Here's how the part is built. I have some questions about the finished solid (model axes, mm). A direction names the side the tool comes from. Give positions to 0.01 mm unless a question says otherwise; leave off trailing zeros. Loops run counter-clockwise (first coordinate to the right, second up) from the corner with the lowest first, then second, coordinate; pieces in that order, holes last.
Q1. Suppose I cut it at B-B (y = 81). List the corners of the cut face in (x, z) for me, and give its area (3 significant figures).
Q2. Suppose I cut it at A-A (y = 19). List the corners of the cut face in (x, z) for me, and give its area (3 significant figures).
Q3. I need wall thicknesses on probe 1 along Y at (x, z) = (3.25, -1.75); probe 2 along Y at (x, z) = (4.25, -3.5) (3 decimals); probe 3 along Z at (x, y) = (0.5, 37.5). Which ranges of each line are inside material? Lowest first, please.
Q4. Thinking about a two-plate mould opening in Z: for faces 4 (the face through (3.493, 83.161, 0.593)), 5 (the face through (3, 20, -6.983)), 6 (the face through (3, 20, 1.017)), 7 (the face through (3.04, 33, -8.75)), which applies, pulls with the +Z half, pulls with the -Z half, needs draft (parallel to the pull), parting line crosses it, or undercut?
Q5. Suppose I cut it at C-C (y = 59.5). List the corners of the cut face in (x, z) for me, and give its area (3 significant figures).
Q6. For faces 1 (the face through (7, 98, -6.755)), 2 (the face through (3, 28.943, -3)), 3 (the face through (7, 98, 0.789)), which set-ups out of +Z, -Z, +X, -X, +Y, -Y let a thin tool reach every point of the face, with its end or its side?
Q7. I'm going to push flat-ended pins straight in: P1, Ø4, axis at y = 77, z = -6, coming from the -X side; P2, Ø2.5, axis at y = 105.83, z = -2.98, coming from the -X side; P3, Ø1.8, axis at x = 3, z = -3, coming from the +Y side; P4, Ø4, axis at x = 5.5, y = 96.5, coming from the +Z side. Where does each tip first touch, or does it pass through?
```python
from build123d import *

# Parameters (mm, degrees)
SKETCH1_R               = 10
SKETCH1_R_2             = 0.8
SKETCH1_R_3             = 3.301767793
BOSS_EXTRUDE1_DEPTH     = 1.5
SKETCH2_R               = 10
BOSS_EXTRUDE2_DEPTH     = 9
CUT_EXTRUDE1_DEPTH      = 93.583714931
CUT_EXTRUDE1_DEPTH_BACK = 93.583714931
SKETCH3_R               = 1.5
FILLET1_R               = 5
SKETCH4_R               = 1.5
BOSS_EXTRUDE3_DEPTH     = 5
CUT_EXTRUDE2_DEPTH      = 4
FILLET3_R               = 2
SKETCH6_W               = 12.069016708
SKETCH6_H               = 36.150412664
BOSS_EXTRUDE4_DEPTH     = 9
CUT_EXTRUDE3_DEPTH      = 112.059195252
CUT_EXTRUDE3_DEPTH_BACK = 112.059195252
CUT_EXTRUDE4_DEPTH      = 111.336877259
CUT_EXTRUDE4_DEPTH_BACK = 111.336877259
SKETCH8_R               = 1
SKETCH8_W               = 8
SKETCH8_H               = 18.5
FILLET4_R               = 4
SKETCH9_W               = 24.382356312
SKETCH9_H               = 35.371587325
CUT_EXTRUDE5_DEPTH      = 3
FILLET5_R               = 4
SKETCH10_R              = 20.065343601
CUT_EXTRUDE6_DEPTH      = 3
CUT_EXTRUDE7_DEPTH      = 111.33687725
CUT_EXTRUDE7_DEPTH_BACK = 111.33687725
FILLET6_R               = 2
CHAMFER1_SIZE           = 3


# Some blends are built 0.0001 mm under size
with BuildPart() as part:
    # Sketch1 → Boss-Extrude1 (new body)
    with BuildSketch(Plane(origin=(0, 0, 0), x_dir=(0, 0, -1), z_dir=(1, 0, 0))):
        with Locations((2.983378847, 10.826778074)):
            Circle(SKETCH1_R)
        with Locations((2.983378847, 18.576778074)):
            Circle(SKETCH1_R_2, mode=Mode.SUBTRACT)
        with Locations((2.983378847, 3.076778074)):
            Circle(SKETCH1_R_2, mode=Mode.SUBTRACT)
        with Locations((-3.266621153, 10.826778074)):
            Circle(SKETCH1_R_2, mode=Mode.SUBTRACT)
        with Locations((9.233378847, 10.826778074)):
            Circle(SKETCH1_R_2, mode=Mode.SUBTRACT)
        with Locations((2.983378847, 10.826778074)):
            Circle(SKETCH1_R_3, mode=Mode.SUBTRACT)
    extrude(amount=BOSS_EXTRUDE1_DEPTH)

    # Sketch2 → Boss-Extrude2 (add)
    with BuildSketch(Plane.ZY):
        with BuildLine():
            Line((-15.531923741, 90.826778074), (9.565166047, 90.826778074))
            Line((9.565166047, 90.826778074), (9.565166047, 10.826778074))
            ThreePointArc((9.565166047, 10.826778074), (-2.983378847, -1.721766821), (-15.531923741, 10.826778074))
            Line((-15.531923741, 10.826778074), (-15.531923741, 90.826778074))
        make_face()
        with Locations((-2.983378847, 10.826778074)):
            Circle(SKETCH2_R, mode=Mode.SUBTRACT)
    extrude(amount=-BOSS_EXTRUDE2_DEPTH)

    # Sketch3 → Cut-Extrude1 (cut, two sides: drawn at the far end of the back side and taken through both)
    with BuildSketch(Plane(origin=(9, 0, 0), x_dir=(0, 0, -1), z_dir=(1, 0, 0)).offset(-CUT_EXTRUDE1_DEPTH_BACK)):
        with Locations((2.983378847, 85.826778074)):
            Circle(SKETCH3_R)
        with BuildLine():
            Line((-3.051129507, 36.150412664), (-3.051129507, 97.572569437))
            Line((-3.051129507, 97.572569437), (-16.389018159, 97.572569437))
            Line((-16.389018159, 97.572569437), (-16.389018159, 8.14109285))
            Line((-16.389018159, 8.14109285), (-9.565166047, 10.826778074))
            add(Edge.make_bspline(
                [(-9.565166047, 10.826778074), (-9.644230884, 15.122204253), (-6.916245701, 23.507010268), (-3.42826878, 31.561714956), (-3.051129507, 36.150412664)],
                knots=[0, 0, 0, 0, 0.482384809, 1, 1, 1, 1], degree=3))
        make_face()
        with BuildLine():
            Line((22.355775853, 8.14109285), (15.531923741, 10.826778074))
            add(Edge.make_bspline(
                [(15.531923741, 10.826778074), (15.610988578, 15.122204253), (12.883003395, 23.507010268), (9.395026474, 31.561714956), (9.017887201, 36.150412664)],
                knots=[0, 0, 0, 0, 0.482384809, 1, 1, 1, 1], degree=3))
            Line((9.017887201, 36.150412664), (9.017887201, 97.572569437))
            Line((9.017887201, 97.572569437), (22.355775853, 97.572569437))
            Line((22.355775853, 97.572569437), (22.355775853, 8.14109285))
        make_face()
    extrude(amount=CUT_EXTRUDE1_DEPTH + CUT_EXTRUDE1_DEPTH_BACK, mode=Mode.SUBTRACT)

    # Fillet1
    fillet1_edges = [part.edges().sort_by_distance(p)[0] for p in [
        (4.5, 90.826778074, 3.051129507),
        (4.5, 90.826778074, -9.017887201),
    ]]
    fillet(fillet1_edges, radius=FILLET1_R)

    # Sketch4 → Boss-Extrude3 (add)
    with BuildSketch(Plane(origin=(9, 0, 0), x_dir=(0, 0, -1), z_dir=(1, 0, 0))):
        with BuildLine():
            Line((-0.788675957, 85.826778074), (-0.788675957, 105.826778074))
            ThreePointArc((-0.788675957, 105.826778074), (2.983378847, 109.598832877), (6.755433651, 105.826778074))
            Line((6.755433651, 105.826778074), (6.755433651, 85.826778074))
            ThreePointArc((6.755433651, 85.826778074), (2.983378847, 82.05472327), (-0.788675957, 85.826778074))
        make_face()
        with Locations((2.983378847, 105.826778074)):
            Circle(SKETCH4_R, mode=Mode.SUBTRACT)
        with Locations((2.983378847, 85.826778074)):
            Circle(SKETCH4_R, mode=Mode.SUBTRACT)
    extrude(amount=-BOSS_EXTRUDE3_DEPTH)

    # Sketch5 → Cut-Extrude2 (cut)
    with BuildSketch(Plane.ZY):
        Polygon((3.051129507, 66.690354093), (-0.520583075, 90.618436978), (8.994411849, 90.618436978), (4.452818785, 66.690354093), align=None)
        Polygon((-9.017887201, 66.690354093), (-5.446174619, 90.618436978), (-12.469802715, 95.280611626), (-31.447569196, 66.690354093), align=None)
    extrude(amount=-CUT_EXTRUDE2_DEPTH, mode=Mode.SUBTRACT)

    # Fillet3
    fillet3_edges = [part.edges().sort_by_distance(p)[0] for p in [
        (2, 90.618436978, -5.446174619),
        (2, 90.618436978, -0.520583075),
    ]]
    fillet(fillet3_edges, radius=FILLET3_R)

    # Sketch6 → Boss-Extrude4 (add)
    with BuildSketch(Plane(origin=(9, 0, 0), x_dir=(0, 0, -1), z_dir=(1, 0, 0))):
        with Locations((2.983378847, 18.075206332)):
            Rectangle(SKETCH6_W, SKETCH6_H)
    extrude(amount=-BOSS_EXTRUDE4_DEPTH)

    # Sketch7 → Cut-Extrude3 (cut, two sides: drawn at the far end of the back side and taken through both)
    with BuildSketch(Plane(origin=(9, 0, 0), x_dir=(0, 0, -1), z_dir=(1, 0, 0)).offset(-CUT_EXTRUDE3_DEPTH_BACK)):
        Polygon((-3.051129507, -1.9847985), (-23.499593466, -1.9847985), (-3.051129507, 36.150412664), (-3.051129507, 6.693164213), (9.017887201, 6.693164213), (9.017887201, 36.150412664), (33.091996179, 2.744303699), (9.017887201, -7.659721138), align=None)
    extrude(amount=CUT_EXTRUDE3_DEPTH + CUT_EXTRUDE3_DEPTH_BACK, mode=Mode.SUBTRACT)

    # Sketch8 → Cut-Extrude4 (cut, two sides: drawn at the far end of the back side and taken through both)
    with BuildSketch(Plane(origin=(9, 0, 0), x_dir=(0, 0, -1), z_dir=(1, 0, 0)).offset(-CUT_EXTRUDE4_DEPTH_BACK)):
        with Locations((2.983378847, 30.648164213)):
            Circle(SKETCH8_R)
        with Locations((2.983378847, 8.738164213)):
            Circle(SKETCH8_R)
        with Locations((2.983378847, 19.693164213)):
            Rectangle(SKETCH8_W, SKETCH8_H)
    extrude(amount=CUT_EXTRUDE4_DEPTH + CUT_EXTRUDE4_DEPTH_BACK, mode=Mode.SUBTRACT)

    # Fillet4
    fillet4_edges = [part.edges().sort_by_distance(p)[0] for p in [
        (4.5, 6.693164213, -9.017887201),
        (4.5, 6.693164213, 3.051129507),
    ]]
    fillet(fillet4_edges, radius=FILLET4_R)

    # Sketch9 → Cut-Extrude5 (cut)
    with BuildSketch(Plane(origin=(9, 0, 0), x_dir=(0, 0, -1), z_dir=(1, 0, 0))):
        with Locations((3.21232116, 16.771571926)):
            Rectangle(SKETCH9_W, SKETCH9_H)
    extrude(amount=-CUT_EXTRUDE5_DEPTH, mode=Mode.SUBTRACT)

    # Fillet5
    # the kernel refuses this fillet: 4 mm, written as the material it takes off along each edge
    with BuildSketch(Plane(origin=(9, 34.457365588, -18.700345567), x_dir=(0, 1, 0), z_dir=(0, 0, 1))) as fillet5_piece_1:
        with BuildLine():
            CenterArc((3.872983346, 4), FILLET5_R, 194.477512186, 75.522487814)
            Line((0, 3), (-0.077459667, 2.98))
            ThreePointArc((-0.077459667, 2.98), (-0.08, 1.5), (-0.08, 0))
            Line((-0.08, 0), (0, -0.08))
            Line((0, -0.08), (3.872983346, -0.08))
            Line((3.872983346, -0.08), (3.872983346, 0))
        make_face()
    extrude(amount=31.43393344, mode=Mode.SUBTRACT)

    # Sketch10 → Cut-Extrude6 (cut)
    with BuildSketch(Plane.ZY):
        with Locations((-2.983378847, 85.826778074)):
            Circle(SKETCH10_R)
    extrude(amount=-CUT_EXTRUDE6_DEPTH, mode=Mode.SUBTRACT)

    # Sketch11 → Cut-Extrude7 (cut, two sides: drawn at the far end of the back side and taken through both)
    with BuildSketch(Plane.ZY.offset(-CUT_EXTRUDE7_DEPTH_BACK)):
        with BuildLine():
            Line((-7.109989343, 76.258566083), (-7.109989343, 35.357320381))
            ThreePointArc((-7.109989343, 35.357320381), (-9.017887201, 33.449422522), (-10.925785059, 35.357320381))
            Line((-10.925785059, 35.357320381), (-10.925785059, 76.258566083))
            ThreePointArc((-10.925785059, 76.258566083), (-9.017887201, 78.166463942), (-7.109989343, 76.258566083))
        make_face()
        with BuildLine():
            Line((1.103749815, 76.258566083), (1.103749815, 35.357320381))
            ThreePointArc((1.103749815, 35.357320381), (3.011647673, 33.449422522), (4.919545531, 35.357320381))
            Line((4.919545531, 35.357320381), (4.919545531, 76.258566083))
            ThreePointArc((4.919545531, 76.258566083), (3.011647673, 78.166463942), (1.103749815, 76.258566083))
        make_face()
    extrude(amount=CUT_EXTRUDE7_DEPTH + CUT_EXTRUDE7_DEPTH_BACK, mode=Mode.SUBTRACT)

    # Fillet6
    fillet6_edges = [part.edges().sort_by_distance(p)[0] for p in [
        (3, 33.449422522, -9.017887201),
        (6.5, 78.166463942, -9.017887201),
        (3, 33.449831083, 3.051129507),
        (6.5, 78.166055381, 3.051129507),
    ]]
    fillet(fillet6_edges, radius=FILLET6_R)

    # Chamfer1
    chamfer1_edges = [part.edges().sort_by_distance(p)[0] for p in [
        (3, 65.761444608, -3.003546718),
    ]]
    chamfer(chamfer1_edges, length=CHAMFER1_SIZE - 0.0001)  # a hair under: the kernel refuses the full size


solid = part.part
```
Solutions:
1. outline: (3, -6.88) - (4, -6.88) - (4, -9.02) - (9, -9.02) - (9, 3.05) - (4, 3.05) - (4, 0.92) - (3, 0.92) - close
1. area: 68.1 mm2
2. outline: (0, -9.02) - (6, -9.02) - (6, -6.98) - (0, -6.98) - close; (0, 1.02) - (6, 1.02) - (6, 3.05) - (0, 3.05) - close
2. area: 24.4 mm2
3. probe 1: y = 6.69 to 10.44, 28.94 to 84.97, 86.68 to 90.76
3. probe 2: y = 6.693 to 7.882, 9.594 to 10.443, 28.943 to 29.792, 31.504 to 84.419, 87.235 to 104.419, 107.235 to 109.563
3. probe 3: z = -7.11 to 1.1
4. face 4: pulls with the +Z half
4. face 5: undercut
4. face 6: undercut
4. face 7: pulls with the -Z half
5. outline: (0, -7.11) - (9, -7.11) - (9, 1.1) - (0, 1.1) - close
5. area: 73.9 mm2
6. face 1: -Z, +X, -X, +Y
6. face 2: +X, -X
6. face 3: +Z, +X, -X, +Y
7. P1: stops at x = 3
7. P2: passes through
7. P3: stops at y = 90.83
7. P4: stops at z = 0.79
